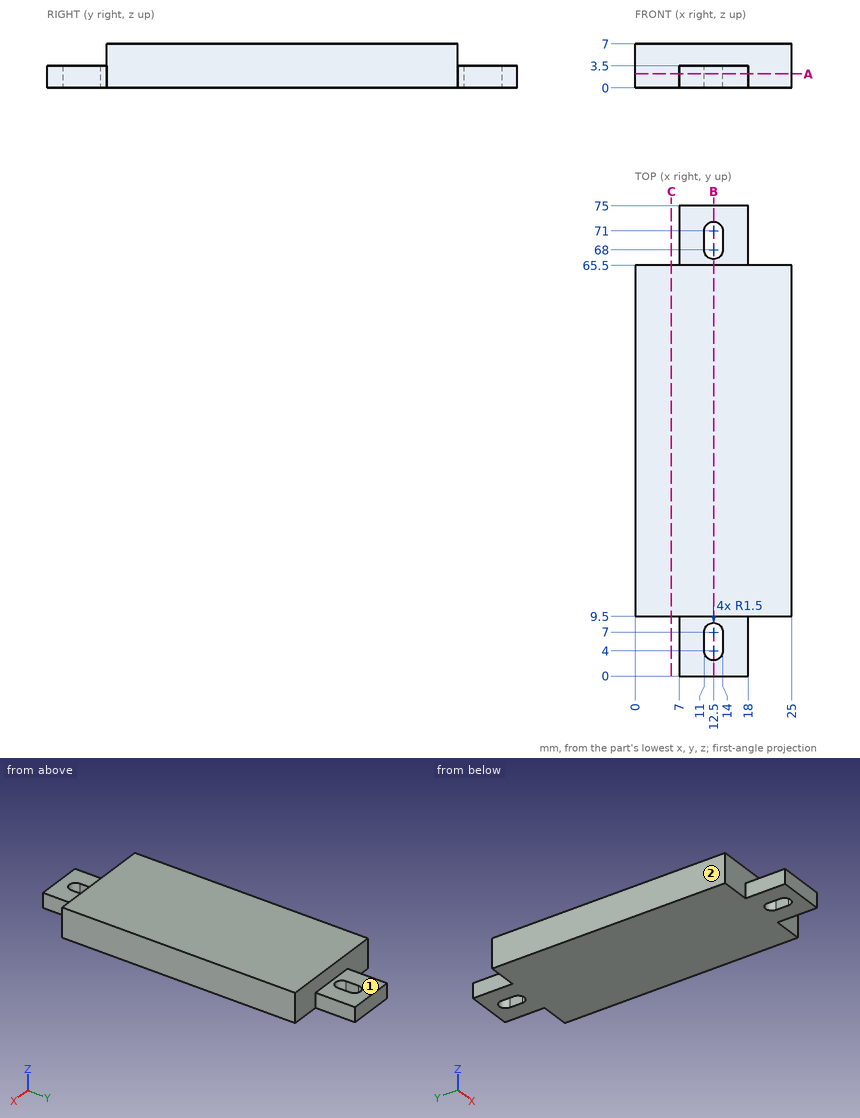
Verification items for this drawing (mm, ordinates from the low corner). A direction names the side the tool comes from. Give positions to 0.01 mm unless a question says otherwise; leave off trailing zeros. Loops run counter-clockwise (first coordinate to the right, second up) from the corner with the lowest first, then second, coordinate; pieces in that order, holes last. Notation, with made-up numbers: M 57,86 L 64,86 A29 ccw 64,115 Z; hole C -3.75,79 d8. An arc over 180 degrees is marked long. Answer as a JSON object with one key per item and string values. Group by question number.
Q1. Material ranges on line 1 along Y through (x, z) = (5.75, 6.5); line 2 along Z through (x, y) = (14.25, 68); line 3 along X through (y, z) = (66, 0.5), recorded low to high. Write a range as [from, to].
Q2. Cross-section at C-C on x = 5.75. Record the cut outline in (y, z), then the cut area to 3 significant figures.
Q3. Cross-section at B-B on x = 12.5. Record the cut outline in (y, z), then the cut area to 4 significant figures.
Q4. Cross-section at A-A on z = 2.25. Record the cut outline in (x, y).
Q5. Go/stop test with flat-tipped pins: P1, Ø0.9, axis at y = 69, z = 1.5, coming from the +X side; P2, Ø3, axis at x = 13, y = 68.5, coming from the +Z side; P3, Ø3.5, axis at y = 5, z = 1.5, coming from the -X side. Record where each tip stops, or that it passes through.
Q6. Access from +Z, -Z, +X, -X, +Y, -Y to the whole of each face (thin tool, end or side, straight path). Record for the marked faces 1 and 2.
Evaluation:
{
 "1": {"line 1": "y = [9.5, 65.5]", "line 2": "z = [0, 3.5]", "line 3": "x = [7, 18]"},
 "2": {"outline": "M 9.5,0 L 65.5,0 L 65.5,7 L 9.5,7 Z", "area": "392 mm2"},
 "3": {"outline": "M 0,0 L 2.5,0 L 2.5,3.5 L 0,3.5 Z; M 8.5,0 L 66.5,0 L 66.5,3.5 L 65.5,3.5 L 65.5,7 L 9.5,7 L 9.5,3.5 L 8.5,3.5 Z; M 72.5,0 L 75,0 L 75,3.5 L 72.5,3.5 Z", "area": "416.5 mm2"},
 "4": {"outline": "M 0,9.5 L 7,9.5 L 7,0 L 18,0 L 18,9.5 L 25,9.5 L 25,65.5 L 18,65.5 L 18,75 L 7,75 L 7,65.5 L 0,65.5 Z; hole M 11,4 A1.5 ccw 14,4 L 14,7 A1.5 ccw 11,7 Z; hole M 11,68 A1.5 ccw 14,68 L 14,71 A1.5 ccw 11,71 Z"},
 "5": {"P1": "stops at x = 18", "P2": "stops at z = 3.5", "P3": "stops at x = 7"},
 "6": {"face 1": "+Z, +X, -X, +Y", "face 2": "+Z, -Z, -X, +Y, -Y"}
}
